from build123d import *

# Parameters (mm, degrees)
SKETCH1_R           = 21
BOSS_EXTRUDE1_DEPTH = 2
SKETCH2_R           = 22.5
BOSS_EXTRUDE2_DEPTH = 1
CUT_EXTRUDE1_DEPTH  = 0.8
CUT_EXTRUDE2_REACH  = 5
SKETCH4_R           = 1.524
SKETCH4_R_2         = 2.8575


with BuildPart() as part:
    # Sketch1 → Boss-Extrude1 (new body)
    with BuildSketch(Plane.XY):
        Circle(SKETCH1_R)
    extrude(amount=BOSS_EXTRUDE1_DEPTH)

    # Sketch2 → Boss-Extrude2 (add)
    with BuildSketch(Plane.XY.offset(2)):
        Circle(SKETCH2_R)
    extrude(amount=BOSS_EXTRUDE2_DEPTH)

    # Sketch3 → Cut-Extrude1 (cut)
    with BuildSketch(Plane(origin=(0, 0, 0), x_dir=(-1, 0, 0), z_dir=(0, 0, -1))):
        with BuildLine():
            Line((15.536569667, 14.527364659), (15.351441673, 14.722858401))
            ThreePointArc((15.351441673, 14.722858401), (12.623062926, 15.941035549), (9.832426491, 14.873161756))
            Line((9.832426491, 14.873161756), (2.990145498, 8.393681964))
            ThreePointArc((2.990145498, 8.393681964), (0.199509062, 7.325808172), (-2.528869685, 8.543985319))
            Line((-2.528869685, 8.543985319), (-9.008349476, 15.386266312))
            ThreePointArc((-9.008349476, 15.386266312), (-11.736728224, 16.604443459), (-14.527364659, 15.536569667))
            Line((-14.527364659, 15.536569667), (-14.722858401, 15.351441673))
            ThreePointArc((-14.722858401, 15.351441673), (-15.941035549, 12.623062926), (-14.873161756, 9.832426491))
            Line((-14.873161756, 9.832426491), (-8.393681964, 2.990145498))
            ThreePointArc((-8.393681964, 2.990145498), (-7.325808172, 0.199509062), (-8.543985319, -2.528869685))
            Line((-8.543985319, -2.528869685), (-15.386266312, -9.008349476))
            ThreePointArc((-15.386266312, -9.008349476), (-16.604443459, -11.736728224), (-15.536569667, -14.527364659))
            Line((-15.536569667, -14.527364659), (-15.351441673, -14.722858401))
            ThreePointArc((-15.351441673, -14.722858401), (-12.623062926, -15.941035549), (-9.832426491, -14.873161756))
            Line((-9.832426491, -14.873161756), (-2.990145498, -8.393681964))
            ThreePointArc((-2.990145498, -8.393681964), (-0.199509062, -7.325808172), (2.528869685, -8.543985319))
            Line((2.528869685, -8.543985319), (9.008349476, -15.386266312))
            ThreePointArc((9.008349476, -15.386266312), (11.736728224, -16.604443459), (14.527364659, -15.536569667))
            Line((14.527364659, -15.536569667), (14.722858401, -15.351441673))
            ThreePointArc((14.722858401, -15.351441673), (15.941035549, -12.623062926), (14.873161756, -9.832426491))
            Line((14.873161756, -9.832426491), (8.393681964, -2.990145498))
            ThreePointArc((8.393681964, -2.990145498), (7.325808172, -0.199509062), (8.543985319, 2.528869685))
            Line((8.543985319, 2.528869685), (15.386266312, 9.008349476))
            ThreePointArc((15.386266312, 9.008349476), (16.604443459, 11.736728224), (15.536569667, 14.527364659))
        make_face()
    extrude(amount=-CUT_EXTRUDE1_DEPTH, mode=Mode.SUBTRACT)

    # Sketch4 → Cut-Extrude2 (cut, up to next)
    with BuildSketch(Plane(origin=(0, 0, 0), x_dir=(-1, 0, 0), z_dir=(0, 0, -1)), mode=Mode.PRIVATE) as cut_extrude2_sk1:
        with Locations((12.402786975, 11.745148679)):
            Circle(SKETCH4_R)
    cut_extrude2_tool1 = extrude(cut_extrude2_sk1.sketch, amount=-CUT_EXTRUDE2_REACH, mode=Mode.PRIVATE) & part.part
    add(cut_extrude2_tool1.solids().sort_by_distance((-12.402787, 11.745149, 0))[0], mode=Mode.SUBTRACT)
    # Sketch4 → Cut-Extrude2 (cut, up to next)
    with BuildSketch(Plane(origin=(0, 0, 0), x_dir=(-1, 0, 0), z_dir=(0, 0, -1)), mode=Mode.PRIVATE) as cut_extrude2_sk2:
        with Locations((11.745148679, -12.402786975)):
            Circle(SKETCH4_R)
    cut_extrude2_tool2 = extrude(cut_extrude2_sk2.sketch, amount=-CUT_EXTRUDE2_REACH, mode=Mode.PRIVATE) & part.part
    add(cut_extrude2_tool2.solids().sort_by_distance((-11.745149, -12.402787, 0))[0], mode=Mode.SUBTRACT)
    # Sketch4 → Cut-Extrude2 (cut, up to next)
    with BuildSketch(Plane(origin=(0, 0, 0), x_dir=(-1, 0, 0), z_dir=(0, 0, -1)), mode=Mode.PRIVATE) as cut_extrude2_sk3:
        with Locations((-12.402786975, -11.745148679)):
            Circle(SKETCH4_R)
    cut_extrude2_tool3 = extrude(cut_extrude2_sk3.sketch, amount=-CUT_EXTRUDE2_REACH, mode=Mode.PRIVATE) & part.part
    add(cut_extrude2_tool3.solids().sort_by_distance((12.402787, -11.745149, 0))[0], mode=Mode.SUBTRACT)
    # Sketch4 → Cut-Extrude2 (cut, up to next)
    with BuildSketch(Plane(origin=(0, 0, 0), x_dir=(-1, 0, 0), z_dir=(0, 0, -1)), mode=Mode.PRIVATE) as cut_extrude2_sk4:
        with Locations((-11.745148679, 12.402786975)):
            Circle(SKETCH4_R)
    cut_extrude2_tool4 = extrude(cut_extrude2_sk4.sketch, amount=-CUT_EXTRUDE2_REACH, mode=Mode.PRIVATE) & part.part
    add(cut_extrude2_tool4.solids().sort_by_distance((11.745149, 12.402787, 0))[0], mode=Mode.SUBTRACT)
    # Sketch4 → Cut-Extrude2 (cut, up to next)
    with BuildSketch(Plane(origin=(0, 0, 0), x_dir=(-1, 0, 0), z_dir=(0, 0, -1)), mode=Mode.PRIVATE) as cut_extrude2_sk5:
        with Locations((6.731624158, -6.374690361)):
            Circle(SKETCH4_R_2)
    cut_extrude2_tool5 = extrude(cut_extrude2_sk5.sketch, amount=-CUT_EXTRUDE2_REACH, mode=Mode.PRIVATE) & part.part
    add(cut_extrude2_tool5.solids().sort_by_distance((-6.731624, -6.37469, 0))[0], mode=Mode.SUBTRACT)
    # Sketch4 → Cut-Extrude2 (cut, up to next)
    with BuildSketch(Plane(origin=(0, 0, 0), x_dir=(-1, 0, 0), z_dir=(0, 0, -1)), mode=Mode.PRIVATE) as cut_extrude2_sk6:
        with Locations((5.501445106, 5.809483862)):
            Circle(SKETCH4_R_2)
    cut_extrude2_tool6 = extrude(cut_extrude2_sk6.sketch, amount=-CUT_EXTRUDE2_REACH, mode=Mode.PRIVATE) & part.part
    add(cut_extrude2_tool6.solids().sort_by_distance((-5.501445, 5.809484, 0))[0], mode=Mode.SUBTRACT)
    # Sketch4 → Cut-Extrude2 (cut, up to next)
    with BuildSketch(Plane(origin=(0, 0, 0), x_dir=(-1, 0, 0), z_dir=(0, 0, -1)), mode=Mode.PRIVATE) as cut_extrude2_sk7:
        with Locations((-5.501445106, -5.809483862)):
            Circle(SKETCH4_R_2)
    cut_extrude2_tool7 = extrude(cut_extrude2_sk7.sketch, amount=-CUT_EXTRUDE2_REACH, mode=Mode.PRIVATE) & part.part
    add(cut_extrude2_tool7.solids().sort_by_distance((5.501445, -5.809484, 0))[0], mode=Mode.SUBTRACT)
    # Sketch4 → Cut-Extrude2 (cut, up to next)
    with BuildSketch(Plane(origin=(0, 0, 0), x_dir=(-1, 0, 0), z_dir=(0, 0, -1)), mode=Mode.PRIVATE) as cut_extrude2_sk8:
        with Locations((-6.731624158, 6.374690361)):
            Circle(SKETCH4_R_2)
    cut_extrude2_tool8 = extrude(cut_extrude2_sk8.sketch, amount=-CUT_EXTRUDE2_REACH, mode=Mode.PRIVATE) & part.part
    add(cut_extrude2_tool8.solids().sort_by_distance((6.731624, 6.37469, 0))[0], mode=Mode.SUBTRACT)
    # Sketch4 → Cut-Extrude2 (cut, up to next)
    with BuildSketch(Plane(origin=(0, 0, 0), x_dir=(-1, 0, 0), z_dir=(0, 0, -1)), mode=Mode.PRIVATE) as cut_extrude2_sk9:
        with BuildLine():
            Line((-11.040615308, 19.604969105), (-5.51854435, 16.261312284))
            ThreePointArc((-5.51854435, 16.261312284), (-3.027783619, 15.183648482), (-0.338986288, 14.815386067))
            Line((-0.338986288, 14.815386067), (0.567529778, 14.815386067))
            ThreePointArc((0.567529778, 14.815386067), (3.210473763, 15.170965551), (5.665462417, 16.212416649))
            Line((5.665462417, 16.212416649), (11.219097888, 19.503380286))
            ThreePointArc((11.219097888, 19.503380286), (0.10268437, 22.499765686), (-11.040615308, 19.604969105))
        make_face()
    cut_extrude2_tool9 = extrude(cut_extrude2_sk9.sketch, amount=-CUT_EXTRUDE2_REACH, mode=Mode.PRIVATE) & part.part
    add(cut_extrude2_tool9.solids().sort_by_distance((-0.08522, 18.896567, 0))[0], mode=Mode.SUBTRACT)


solid = part.part
Read the model definition and answer for the solid it produces. Units are mm, in the model's axes. A direction names the side the tool comes from. Coordinates: 2 decimals unless noted, no trailing zeros. Loops run counter-clockwise (first coordinate to the right, second up) from the corner with the lowest first, then second, coordinate; pieces in that order, holes last.
Q1. The part is cut by section A-A on z = 1.35. Give the number of separate pieces and of enclosed holes in the cut face, and give its area (3 significant figures).
Q2. The mould has two halves that part along X. Classify faces 1 (the face through (16, 1, 0)), 2 (the face through (-11.917, 5.723, 0.394)), 3 (the face through (15.883, 11.836, 0.394)), 4 (the face through (-0.72, -22.49, 2.49)): +X half, -X half, draft (parallel to the pull), parting line (faces both ways), or undercut.
Q3. Each of these flat-tipped pins is pushed along its axis until it touches: pin 1 Ø4 at (x, y) = (2.5, 3) entering from -Z; pin 2 Ø12.5 at (x, y) = (-0.5, 6.5) entering from -Z; pin 3 Ø5 at (x, y) = (-5.5, 5.81) entering from -Z. Where does it stop, or does it pass through?
Q4. The part is cut by section B-B on x = 1.5. Write down the section's boundary in (y, z).
Q5. The part is cut by section D-D on x = -18. Write down the section's boundary in (y, z), and give its area (3 significant figures).
Q6. Consider probe 1 along X at (y, z) = (-13, 2.55); probe 2 along X at (y, z) = (8, 1.7); probe 3 along Z at (x, y) = (-14.5, 11.5). Determine where each line is inside the solid, lowest interval first.
Q7. The part is cut by section C-C on y = 0. Write down the section's boundary in (x, z), and give its area (3 significant figures).
Q8. Which of the six approach directions +Z, -Z, +X, -X, +Y, -Y give full straight-line access (tool end or side, diameter ignored) to faces 5 (the face through (12.601, -10.234, 1.885)), 6 (the face through (0, 0, 0.8)), 7 (the face through (-7.79, 17.47, 1.48))?
Results below:
1. separate pieces: 1
1. enclosed holes: 8
1. area: 1,180 mm2
2. face 1: draft
2. face 2: undercut
2. face 3: undercut
2. face 4: parting line
3. pin 1: stops at z = 0.8
3. pin 2: stops at z = 0
3. pin 3: passes through
4. outline: (-22.45, 2) - (-20.95, 2) - (-20.95, 0) - (-7.51, 0) - (-7.51, 0.8) - (7.77, 0.8) - (7.77, 0) - (14.88, 0) - (14.88, 3) - (-22.45, 3) - close
5. outline: (-13.5, 2) - (-10.82, 2) - (-10.82, 0) - (10.82, 0) - (10.82, 2) - (13.5, 2) - (13.5, 3) - (-13.5, 3) - close
5. area: 70.3 mm2
6. probe 1: x = -18.36 to -13.15, -10.34 to 11.54, 13.27 to 18.36
6. probe 2: x = -19.42 to -7.34, -3.67 to 4.38, 9.08 to 19.42
6. probe 3: z = 0.8 to 3
7. outline: (-22.5, 2) - (-21, 2) - (-21, 0) - (-7.34, 0) - (-7.34, 0.8) - (7.34, 0.8) - (7.34, 0) - (21, 0) - (21, 2) - (22.5, 2) - (22.5, 3) - (-22.5, 3) - close
7. area: 117 mm2
8. face 5: +Z, -Z
8. face 6: -Z
8. face 7: +Z, -Z, +Y
